```python
from build123d import *

# Parameters (mm, degrees)
HOLE_WIZARD_M3_1_D       = 2.5
HOLE_WIZARD_M2_5_1_D     = 2.05
HOLE_WIZARD_M2_5_1_DEPTH = 3.75
HOLE_WIZARD_M2_5_1_TIP   = 0.615882135
CHAMFER_1_SIZE           = 0.3
MM_1_D                   = 3
MM_1_DEPTH               = 10
MM_1_TIP                 = 0.901290929


with BuildPart() as part:
    # Sketch 1 → Revolve 1 (revolve)
    with BuildSketch(Plane.XY, mode=Mode.PRIVATE) as revolve_1_sk:
        Polygon((0, 0), (0, 2.5), (4, 2.5), (4, 3), (23.4, 3), (23.4, 9), (26.4, 9), (26.4, 3), (30.4, 3), (30.4, 2.5), (34.4, 2.5), (34.4, 0), align=None)
    revolve(revolve_1_sk.sketch.rotate(Axis((34.4, 0, 0), (-1, 0, 0)), 90), axis=Axis((34.4, 0, 0), (-1, 0, 0)))

    # Hole Wizard M3 _1 (through all)
    with Locations(Plane(origin=(26.4, 4.949747468, 4.949747468), x_dir=(0, 0, 1), z_dir=(1, 0, 0))):
        with Locations((0, 0), (-9.899494936, 0), (-9.899494936, 9.899494936), (0, 9.899494936)):
            Hole(HOLE_WIZARD_M3_1_D / 2)

    # Hole Wizard M2.5 _1
    with Locations(Plane(origin=(28.4, 3, 0), x_dir=(0, 0, 1), z_dir=(0, 1, 0))):
        with Locations((0, 0)):
            Hole(HOLE_WIZARD_M2_5_1_D / 2, depth=HOLE_WIZARD_M2_5_1_DEPTH)
            with Locations((0, 0, -(HOLE_WIZARD_M2_5_1_DEPTH + HOLE_WIZARD_M2_5_1_TIP / 2))):  # 118° drill point
                Cone(0, HOLE_WIZARD_M2_5_1_D / 2, HOLE_WIZARD_M2_5_1_TIP, mode=Mode.SUBTRACT)

    # Chamfer 1
    chamfer_1_edges = [part.edges().sort_by_distance(p)[0] for p in [
        (26.4, 0, 9),
        (0, 0, 2.5),
        (34.4, 0, 2.5),
    ]]
    chamfer(chamfer_1_edges, length=CHAMFER_1_SIZE)

    # mm _1
    with Locations(Plane(origin=(34.4, 0, 0), x_dir=(0, 0, 1), z_dir=(1, 0, 0))):
        with Locations((0, 0)):
            Hole(MM_1_D / 2, depth=MM_1_DEPTH)
            with Locations((0, 0, -(MM_1_DEPTH + MM_1_TIP / 2))):  # 118° drill point
                Cone(0, MM_1_D / 2, MM_1_TIP, mode=Mode.SUBTRACT)


solid = part.part
```
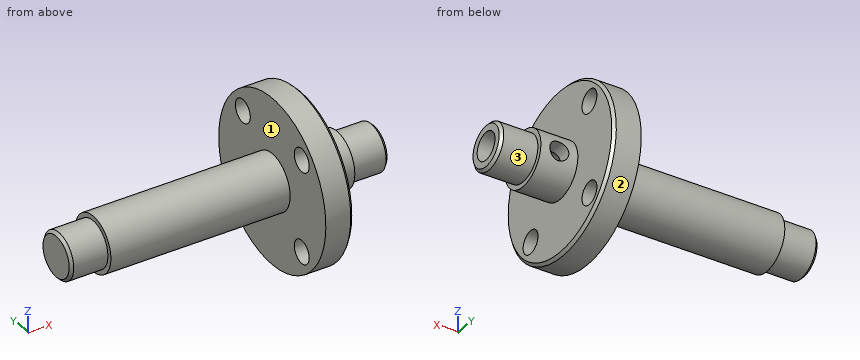
For this review, take the finished solid that the model builds, in its own axes (mm). Face numbers are marked on the shaded views. A direction names the side the tool comes from. Coordinates: 2 decimals unless noted, no trailing zeros. Write each loop counter-clockwise with the first axis right and the second up, starting at its lowest first coordinate (ties: lowest second). Pieces come first, ordered by that corner, then holes.
(1) Add section B-B on x = 21. Give the boundary of the cut face in (y, z), then the cut area to 3 significant figures.
(2) Add section A-A on x = 27. Give the boundary of the cut face in (y, z).
(3) Tool access review of the marked faces 1, 2 and 3: name each direction out of +Z, -Z, +X, -X, +Y, -Y from which nothing blocks a thin tool from reaching the whole face with its end or side.
(4) For pin 1 Ø6 at (y, z) = (4, -2) entering from -X; pin 2 Ø6 at (y, z) = (-5, -3) entering from -X; pin 3 Ø4 at (x, y) = (3.5, 6) entering from -Z; pin 4 Ø3 at (y, z) = (4.95, 4.95) entering from -X, all flat-tipped, find the tip position at first contact; note any pin that passes through.
(5) Wall thickness on probe 1 along X at (y, z) = (2.05, 0) (3 decimals); probe 2 along X at (y, z) = (7, -4.75); probe 3 along Y at (x, z) = (23.5, -5.75): over which ranges is each line inside the solid? List them lowest first.
(6) Add section C-C on z = 5.5. Count the separate pieces of the cut face and the enclosed holes in it, then the cut area to 3 significant figures.
Answer sheet:
1. outline: circle Ø6 at (0, 0)
1. area: 28.3 mm2
2. outline: circle Ø6 at (0, 0); hole circle Ø3 at (0, 0)
3. face 1: -X
3. face 2: +X, -X
3. face 3: +X
4. pin 1: stops at x = 0
4. pin 2: stops at x = 4
4. pin 3: passes through
4. pin 4: stops at x = 23.4
5. probe 1: x = 0 to 27.375, 29.425 to 34.4
5. probe 2: x = 23.4 to 26.4
5. probe 3: y = -6.92 to -5.91, -3.99 to 3.99, 5.91 to 6.92
6. separate pieces: 3
6. enclosed holes: 0
6. area: 29.2 mm2
